Read the model definition and answer for the solid it produces. Units are mm, in the model's axes. Round coordinates to 2 decimals unless told otherwise and drop trailing zeros. Loops run counter-clockwise (first coordinate to the right, second up) from the corner with the lowest first, then second, coordinate; pieces in that order, holes last. Notation, with made-up numbers: M 53.5,5.5 L 84.5,5.5 A25 cw 84.5,34.5 Z; hole C 20.25,21.25 d11. An arc over 180 degrees is marked long. Write each question's results on one line, items separated by ' | '.
from build123d import *

# Parameters (mm, degrees)
F0_R           = 32
F1_DEPTH       = 10
F3_D           = 3.3
F3_CSINK_D     = 6.72
F3_CSINK_ANGLE = 90
F5_D           = 3.3
F5_CSINK_D     = 6.72
F5_CSINK_ANGLE = 90
F6_R           = 11.5
F7_DEPTH       = 10.001
F9_DEPTH       = 32.001
F9_DEPTH_BACK  = 32.001


with BuildPart() as f1:
    # F0 (on Right) → F1 (new body)
    with BuildSketch(Plane.YZ):
        Circle(F0_R)
    extrude(amount=F1_DEPTH)

    # F3 (through all)
    with Locations(Plane.YZ.offset(10)):
        with Locations((-13, 13), (13, 13), (13, -13), (-13, -13)):
            CounterSinkHole(F3_D / 2, F3_CSINK_D / 2, counter_sink_angle=F3_CSINK_ANGLE)

    # F5 (through all)
    with Locations(Plane.YZ.offset(10)):
        with Locations((-7, 24.7), (7, 24.7), (-7, -24.7), (7, -24.7)):
            CounterSinkHole(F5_D / 2, F5_CSINK_D / 2, counter_sink_angle=F5_CSINK_ANGLE)

    # F6 (on face) → F7 (cut, through all)
    with BuildSketch(Plane.YZ.offset(10)):
        Circle(F6_R)
    extrude(amount=-F7_DEPTH, mode=Mode.SUBTRACT)

    # F8 (on Top) → F9 (cut, two sides)
    with BuildSketch(Plane.XY) as f9_sk:
        Polygon((0, -25), (0, -32), (7, -32), align=None)
        Polygon((0, 32), (0, 25), (7, 32), align=None)
    extrude(amount=-F9_DEPTH, mode=Mode.SUBTRACT)
    extrude(f9_sk.sketch, amount=F9_DEPTH_BACK, mode=Mode.SUBTRACT)


solid = f1.part
Item 1: Straight lines are drawn through the part: line 1 (Z direction, x = 4.25, y = 7); line 2 (Z direction, x = 1, y = -13.5); line 3 (Z direction, x = 2, y = -13). For each, find the intervals that lie inside material, in ascending order.
Outcome:
line 1: z = -31.22 to -26.35, -23.05 to -9.12, 9.12 to 23.05, 26.35 to 31.22 | line 2: z = -29.01 to -14.57, -11.43 to 11.43, 14.57 to 29.01 | line 3: z = -29.24 to -14.65, -11.35 to 11.35, 14.65 to 29.24
Item 2: The mould has two halves that part along Y. Classify faces 1 (the face through (3, 28, 0)), 2 (the face through (4.087, 11.476, 12.368)), 3 (the face through (7.15, -31.97, 1.41)): pulls with the +Y half, pulls with the -Y half, needs draft (parallel to the pull), parting line crosses it, or undercut.
Outcome:
face 1: pulls with the +Y half | face 2: undercut | face 3: parting line crosses it
Item 3: Flat-ended cylindrical pins translate along their axes: pin 1 (4 mm diameter, centred on x = 6.5, z = -5.5, fed in from -Y); pin 2 (4.5 mm diameter, centred on y = 7, z = 24.7, fed in from +X); pin 3 (4 mm diameter, centred on y = -7, z = 24.7, fed in from +X). Find the tip coordinate at first contact, or state that the pin passes through.
Outcome:
pin 1: stops at y = -31.81 | pin 2: stops at x = 8.89 | pin 3: stops at x = 8.64
Item 4: The part is cut by section B-B (y = 0). Determine the outline of the cut face in (x, z), plus the area to 3 significant figures.
Outcome:
outline: M 0,-32 L 10,-32 L 10,-11.5 L 0,-11.5 Z; M 0,11.5 L 10,11.5 L 10,32 L 0,32 Z | area: 410 mm2
Item 5: The part is cut by section C-C (x = 4). State how many separate pieces and enclosed holes the cut face has, plus the area to 3 significant figures.
Outcome:
separate pieces: 1 | enclosed holes: 9 | area: 2,620 mm2
Item 6: The part is cut by section D-D (y = 13). Determine the outline of the cut face in (x, z), plus the area to 3 significant figures.
Outcome:
outline: M 0,-29.24 L 10,-29.24 L 10,-16.36 L 8.29,-14.65 L 0,-14.65 Z; M 0,-11.35 L 8.29,-11.35 L 10,-9.64 L 10,9.64 L 8.29,11.35 L 0,11.35 Z; M 0,14.65 L 8.29,14.65 L 10,16.36 L 10,29.24 L 0,29.24 Z | area: 513 mm2
Item 7: The part is cut by section A-A (z = 0). Determine the outline of the cut face in (x, y), plus the area to 3 significant figures.
Outcome:
outline: M 0,-25 L 7,-32 L 10,-32 L 10,-11.5 L 0,-11.5 Z; M 0,11.5 L 10,11.5 L 10,32 L 7,32 L 0,25 Z | area: 361 mm2
